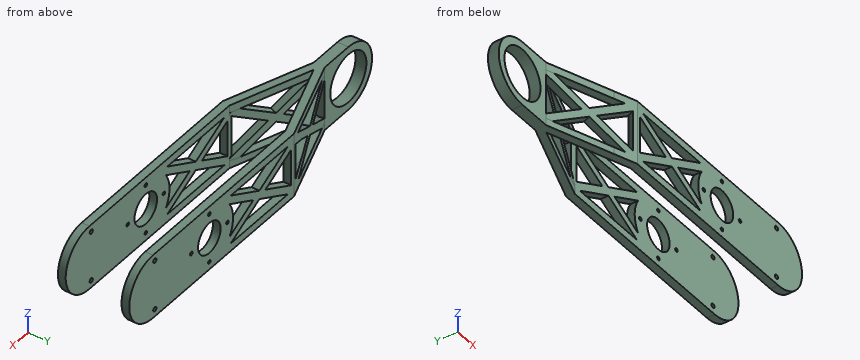
from build123d import *

# Parameters (mm, degrees)
SKETCH_1_R               = 21
SKETCH_1_R_2             = 16
EXTRUDE_1_DEPTH          = 46
SKETCH_1_R_3             = 10
EXTRUDE_1_2_DEPTH        = 46
SKETCH_2_W               = 150
SKETCH_2_H               = 5
EXTRUDE_3_DEPTH          = 5
SKETCH_3_W               = 150
SKETCH_3_H               = 5
EXTRUDE_4_DEPTH          = 5
EXTRUDE_5_DEPTH          = 5
SKETCH_6_W               = 169.409921662
SKETCH_6_H               = 36
CUT_EXTRUDE_1_DEPTH      = 42
CUT_EXTRUDE_4_REACH      = 155.15
EXTRUDE_7_DEPTH          = 5
EXTRUDE_8_REACH          = 155.15
EXTRUDE_8_END_RADIUS     = 21
SKETCH_10_W              = 21
SKETCH_10_H              = 7
SKETCH_11_W              = 54.75
SKETCH_11_H              = 32.4550301
CUT_EXTRUDE_5_DEPTH      = 5
EXTRUDE_15_DEPTH         = 5
SKETCH_13_R              = 1.125
CUT_EXTRUDE_6_DEPTH      = 150.607304507
CUT_EXTRUDE_6_DEPTH_BACK = 150.607304507
SKETCH_14_R              = 1.4
CUT_EXTRUDE_7_DEPTH      = 150.607304507
CUT_EXTRUDE_7_DEPTH_BACK = 150.607304507


with BuildPart() as part:
    # Sketch 1 → Extrude 1 (new body)
    with BuildSketch(Plane(origin=(0, 0, 0), x_dir=(1, 0, 0), z_dir=(0, 1, 0))):
        with Locations(Location((-81.089427727, -5.294054995, 0), (0, 0, 270))):
            Circle(SKETCH_1_R)
        with Locations(Location((-81.089427727, -5.294054995, 0), (0, 0, 270))):
            Circle(SKETCH_1_R_2, mode=Mode.SUBTRACT)
    extrude(amount=EXTRUDE_1_DEPTH)



with BuildPart() as body_2:
    # Sketch 1 → Extrude 1 2 (new body)
    with BuildSketch(Plane(origin=(0, 0, 0), x_dir=(1, 0, 0), z_dir=(0, 1, 0))):
        with BuildLine():
            Line((68.910572273, 15.705945005), (118.910572273, 15.705945005))
            ThreePointArc((118.910572273, 15.705945005), (139.910572273, -5.294054995), (118.910572273, -26.294054995))
            Line((118.910572273, -26.294054995), (68.910572273, -26.294054995))
            ThreePointArc((68.910572273, -26.294054995), (47.910572273, -5.294054995), (68.910572273, 15.705945005))
        make_face()
        with Locations(Location((68.910572273, -5.294054995, 0), (0, 0, 270))):
            Circle(SKETCH_1_R_3, mode=Mode.SUBTRACT)
    extrude(amount=EXTRUDE_1_2_DEPTH)


with BuildPart() as part_1:
    add(part.part)

    add(body_2.part)  # Extrude 3 merges body 2
    # Sketch 2 → Extrude 3 (add)
    with BuildSketch(Plane(origin=(0, 46, 0), x_dir=(1, 0, 0), z_dir=(0, 1, 0))):
        with Locations((-6.089427727, -23.794054995)):
            Rectangle(SKETCH_2_W, SKETCH_2_H)
        with Locations((-6.089427727, 13.205945005)):
            Rectangle(SKETCH_2_W, SKETCH_2_H)
    extrude(amount=-EXTRUDE_3_DEPTH)

    # Sketch 3 → Extrude 4 (add)
    with BuildSketch(Plane.XZ):
        with Locations((-6.089427727, -13.205945005)):
            Rectangle(SKETCH_3_W, SKETCH_3_H)
        with Locations((-6.089427727, 23.794054995)):
            Rectangle(SKETCH_3_W, SKETCH_3_H)
    extrude(amount=-EXTRUDE_4_DEPTH)

    # Sketch 4 → Extrude 5 (add)
    with BuildSketch(Plane.XZ):
        Polygon((-36.788692473, 8.113223678), (-7.244877213, 23.511020598), (-6.089427727, 21.294054995), (-4.933978242, 23.511020598), (24.609837018, 8.113223678), (54.153652279, 23.511020598), (56.46455125, 19.077089392), (30.018987378, 5.294054995), (56.46455125, -8.488979402), (54.153652279, -12.922910608), (24.609837018, 2.474886312), (-4.933978242, -12.922910608), (-7.244877213, -12.922910608), (-36.788692473, 2.474886312), (-66.332507733, -12.922910608), (-68.643406704, -8.488979402), (-42.197842833, 5.294054995), (-68.643406704, 19.077089392), (-66.332507733, 23.511020598), align=None)
        Polygon((-31.379542113, 5.294054995), (-8.589427727, -6.583813521), (-8.589427727, 17.17192351), align=None, mode=Mode.SUBTRACT)
        Polygon((-3.589427727, -6.583813521), (19.200686659, 5.294054995), (-3.589427727, 17.17192351), align=None, mode=Mode.SUBTRACT)
    extrude_5 = extrude(amount=-EXTRUDE_5_DEPTH)

    # Sketch 6 → Cut-Extrude 1 (cut)
    with BuildSketch(Plane(origin=(0, 0, -15.705945005), x_dir=(-1, 0, 0), z_dir=(0, 0, -1))):
        with Locations((-75.35345041, 23)):
            Rectangle(SKETCH_6_W, SKETCH_6_H)
    extrude(amount=-CUT_EXTRUDE_1_DEPTH, mode=Mode.SUBTRACT)

    # Mirror 1: Extrude 5 across plane
    add(extrude_5.mirror(Plane.ZX.offset(23)))

    # Cut-Extrude 4: up to this face of the body (flat: up to its plane)
    cut_extrude_4_end = Plane(part_1.part.faces().sort_by_distance((18.910572273, 43.5, 26.294054995))[0])
    # Sketch 7 → Cut-Extrude 4 (cut, up to the picked face)
    with BuildSketch(Plane(origin=(0, 0, -15.705945005), x_dir=(-1, 0, 0), z_dir=(0, 0, -1)), mode=Mode.PRIVATE) as cut_extrude_4_sk1:
        Polygon((6.089427727, 0), (60.089427727, 19.5), (108.089427727, 19.5), (108.089427727, 26.5), (60.089427727, 26.5), (6.089427727, 46), (127.814090618, 46), (127.814090618, 0), align=None)
    cut_extrude_4_tool1 = split(extrude(cut_extrude_4_sk1.sketch, amount=-CUT_EXTRUDE_4_REACH, mode=Mode.PRIVATE), bisect_by=cut_extrude_4_end, keep=Keep.BOTH, mode=Mode.PRIVATE)
    add(cut_extrude_4_tool1.solids().sort_by(Axis((-33.531395, 8.526091, -15.705945), (0, 0, 1)))[0], mode=Mode.SUBTRACT)


with BuildPart() as cut_extrude_4_piece_1:
    # of the separate pieces the step leaves, piece 1, a body of its own (cut_extrude_4_pieces)
    add(part_1.part.solids().sort_by_distance((-6.089427727, 0, -15.705945005))[0])



with BuildPart() as cut_extrude_4_piece_2:
    # of the separate pieces the step leaves, piece 2, a body of its own (cut_extrude_4_pieces)
    add(part_1.part.solids().sort_by_distance((118.910572273, 41, 26.294054995))[0])


with BuildPart() as cut_extrude_4_piece_3:
    # of the separate pieces the step leaves, piece 3, a body of its own (cut_extrude_4_pieces)
    add(part_1.part.solids().sort_by_distance((-81.089427727, 19.5, 26.294054995))[0])


with BuildPart() as cut_extrude_4_piece_1_1:
    add(cut_extrude_4_piece_1.part)

    add(cut_extrude_4_piece_2.part)  # Extrude 7 merges Cut-Extrude 4 piece 2

    add(cut_extrude_4_piece_3.part)  # Extrude 7 merges Cut-Extrude 4 piece 3
    # Sketch 9 → Extrude 7 (add)
    with BuildSketch(Plane(origin=(0, 0, -15.705945005), x_dir=(-1, 0, 0), z_dir=(0, 0, -1))):
        Polygon((4.391205408, 41.297230502), (55.060459105, 23), (4.391205408, 4.702769498), (6.089427727, 0), (69.781735419, 23), (6.089427727, 46), align=None)
    extrude_7 = extrude(amount=-EXTRUDE_7_DEPTH)

    # Extrude 8: up to this cylinder (the profile starts outside it)
    extrude_8_end = Plane(origin=(-81.089427727, 23, 5.294054995), z_dir=(0, -1, 0)) * Cylinder(EXTRUDE_8_END_RADIUS, 353.3, mode=Mode.PRIVATE)
    # Sketch 10 → Extrude 8 (add, up to the surface)
    with BuildSketch(Plane(origin=(0, 0, -15.705945005), x_dir=(-1, 0, 0), z_dir=(0, 0, -1)), mode=Mode.PRIVATE) as extrude_8_sk1:
        with Locations((70.589427727, 23)):
            Rectangle(SKETCH_10_W, SKETCH_10_H)
    extrude_8_tool1 = extrude(extrude_8_sk1.sketch, amount=-EXTRUDE_8_REACH, mode=Mode.PRIVATE) - extrude_8_end
    extrude_8 = extrude_8_tool1.solids().sort_by_distance((-70.589428, 23, -15.705945))[0]
    add(extrude_8)

    # Mirror 2: Extrude 7, Extrude 8 across plane
    add(extrude_7.mirror(Plane(origin=(0, 0, 5.294054995), x_dir=(1, 0, 0), z_dir=(0, 0, -1))))
    add(extrude_8.mirror(Plane(origin=(0, 0, 5.294054995), x_dir=(1, 0, 0), z_dir=(0, 0, -1))))

    # Sketch 11 → Cut-Extrude 5 (cut)
    with BuildSketch(Plane(origin=(-0.702466407, -1.945291588, 0), x_dir=(0.9405538996916954, -0.3396444637775568, 0), z_dir=(-0.3396444637775568, -0.9405538996916956, 0))):
        with Locations((-35.765412623, 5.066539945)):
            Rectangle(SKETCH_11_W, SKETCH_11_H)
    extrude(amount=-CUT_EXTRUDE_5_DEPTH, mode=Mode.SUBTRACT)

    # Sketch 12 → Extrude 15 (add)
    with BuildSketch(Plane(origin=(-0.702466407, -1.945291588, 0), x_dir=(0.9405538996916956, -0.33964446377755675, 0), z_dir=(-0.33964446377755675, -0.9405538996916956, 0))):
        Polygon((-31.030335125, 5.165890673), (-6.246195793, -9.525798606), (-8.795823184, -13.826891509), (-35.96762349, 2.280169619), (-64.18375705, -14.211451822), (-66.706787961, -9.894703622), (-40.887006083, 5.196310444), (-66.473080759, 20.363375718), (-63.923453368, 24.664468621), (-35.949717718, 8.082031497), (-8.84109266, 23.926342034), (-6.318061748, 19.609593834), align=None)
    extrude_15 = extrude(amount=-EXTRUDE_15_DEPTH)

    # Mirror 3: Extrude 15 across plane
    add(extrude_15.mirror(Plane.ZX.offset(23)))

    # Sketch 13 → Cut-Extrude 6 (cut, two sides)
    with BuildSketch(Plane(origin=(0, 46, 0), x_dir=(1, 0, 0), z_dir=(0, 1, 0))) as cut_extrude_6_sk:
        with Locations(Location((84.910572273, -5.294054995, 0), (0, 0, 270))):
            Circle(SKETCH_13_R)
        with Locations(Location((52.910572273, -5.294054995, 0), (0, 0, 270))):
            Circle(SKETCH_13_R)
        with Locations(Location((68.910572273, -21.294054995, 0), (0, 0, 270))):
            Circle(SKETCH_13_R)
        with Locations(Location((68.910572273, 10.705945005, 0), (0, 0, 270))):
            Circle(SKETCH_13_R)
    extrude(amount=CUT_EXTRUDE_6_DEPTH, mode=Mode.SUBTRACT)
    extrude(cut_extrude_6_sk.sketch, amount=-CUT_EXTRUDE_6_DEPTH_BACK, mode=Mode.SUBTRACT)

    # Sketch 14 → Cut-Extrude 7 (cut, two sides)
    with BuildSketch(Plane(origin=(0, 46, 0), x_dir=(1, 0, 0), z_dir=(0, 1, 0))) as cut_extrude_7_sk:
        with Locations(Location((117.277150097, 10.955945005, 0), (0, 0, 270))):
            Circle(SKETCH_14_R)
        with Locations(Location((117.277150097, -21.544054995, 0), (0, 0, 270))):
            Circle(SKETCH_14_R)
    extrude(amount=CUT_EXTRUDE_7_DEPTH, mode=Mode.SUBTRACT)
    extrude(cut_extrude_7_sk.sketch, amount=-CUT_EXTRUDE_7_DEPTH_BACK, mode=Mode.SUBTRACT)


solid = cut_extrude_4_piece_1_1.part
The model under review builds one solid part; all positions refer to its coordinate system, in mm. Give positions to 0.01 mm unless a question says otherwise; leave off trailing zeros. Order: outer loops, then holes, each group sorted by start corner. A loop starts at its lowest first (then second) coordinate and runs counter-clockwise, first axis right, second up. Notation, with made-up numbers: M 28.25,88.5 L 36.25,88.5 A20 cw 36.25,120.5 Z; hole C 87.25,42.5 d2. An arc over 180 degrees is marked long. Use one line per item in the form item = value. Start each with the question number.
Item 1: We need section B-B on x = 36.5. Give the number of separate pieces and of enclosed holes in the cut face, plus the area to 3 significant figures.
Item 2: Insertion check: pin 1 Ø1.3 at (x, z) = (52.91, 5.29) entering from +Y; pin 2 Ø5 at (x, z) = (-31.5, -8.5) entering from +Y; pin 3 Ø2.5 at (y, z) = (3, 10) entering from +X; pin 4 Ø5.5 at (y, z) = (23.5, 7) entering from +X. Each pin has a flat end and moves straight along its axis. Give the tip position at first contact, or say it passes through.
Item 3: We need section A-A on x = 96. Give the boundary of the cut face in (y, z), plus the area to 3 significant figures.
Item 4: To check wall thickness, follow line 1 along Y through (x, z) = (4, 17); line 2 along X through (y, z) = (24, 5); line 3 along Y through (x, z) = (-81, 23.5). State the ranges of each line that lie inside material, in increasing order. Write a range as from..to.
Completed:
q1.separate_pieces = 8
q1.enclosed_holes = 0
q1.area = 213 mm²
q2.pin_1 = through
q2.pin_2 = 37.25
q2.pin_3 = 139.62
q2.pin_4 = -60.09
q3.outline = M 0,-15.71 L 5,-15.71 L 5,26.29 L 0,26.29 Z; M 41,-15.71 L 46,-15.71 L 46,26.29 L 41,26.29 Z
q3.area = 420 mm²
q4.line_1 = 0..5, 41..46
q4.line_2 = -102.09..-97.09, -65.09..-60.09
q4.line_3 = 19.5..26.5
